from build123d import *

# Parameters (mm, degrees)
SKETCH_1_W      = 83.5
SKETCH_1_H      = 83.5
SKETCH_1_W_2    = 77.5
SKETCH_1_H_2    = 77.5
EXTRUDE_1_DEPTH = 20
CHAMFER_1_SIZE  = 1.5
SKETCH_2_W      = 83.5
SKETCH_2_H      = 83.5
EXTRUDE_2_DEPTH = 3


with BuildPart() as part:
    # Эскиз1 → Бобышка-Вытянуть1 (new body)
    with BuildSketch(Plane.XY):
        with Locations((38.75, 38.75)):
            Rectangle(SKETCH_1_W, SKETCH_1_H)
        with Locations((38.75, 38.75)):
            Rectangle(SKETCH_1_W_2, SKETCH_1_H_2, mode=Mode.SUBTRACT)
    extrude(amount=EXTRUDE_1_DEPTH)

    # Фаска1
    chamfer_1_edges = [part.edges().sort_by_distance(p)[0] for p in [
        (0, 38.75, 0),
        (38.75, 0, 0),
        (77.5, 38.75, 0),
        (38.75, 77.5, 0),
    ]]
    chamfer(chamfer_1_edges, length=CHAMFER_1_SIZE)

    # Эскиз2 → Бобышка-Вытянуть2 (add)
    with BuildSketch(Plane.XY.offset(20)):
        with Locations((38.75, 38.75)):
            Rectangle(SKETCH_2_W, SKETCH_2_H)
    extrude(amount=EXTRUDE_2_DEPTH)


solid = part.part
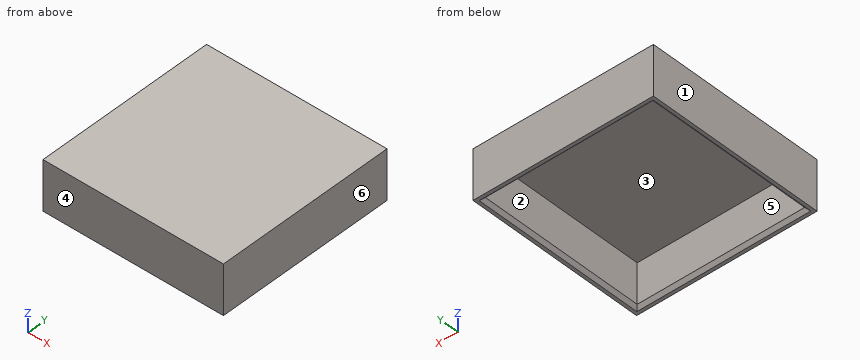
Input: part model. Units: mm. Frame: model coordinates. Face numbers are marked on the shaded views. A direction names the side the tool comes from. Coordinates: 2 decimals unless noted, no trailing zeros. Order: outer loops, then holes, each group sorted by start corner. A loop starts at its lowest first (then second) coordinate and runs counter-clockwise, first axis right, second up. Notation, with made-up numbers: M 29.5,56.25 L 50.5,56.25 A19 ccw 50.5,66.25 Z; hole C -37.75,30.5 d1. An arc over 180 degrees is marked long. Answer in a Markdown table with one row per item.
(1) Section query B-B, the plane z = 15.25. Output: boundary loops of the cut face in (x, y), plus the area to 3 significant figures.
Numbers:
| item | result |
|---|---|
| outline | M -3,-3 L 80.5,-3 L 80.5,80.5 L -3,80.5 Z; hole M 0,0 L 77.5,0 L 77.5,77.5 L 0,77.5 Z |
| area | 966 mm^2 |
(2) Contact query for a flat-ended pin moving along its axis: pin 1 Ø23 at (x, y) = (36, 52.5) entering from -Z. Output: stop coordinate, or through.
Numbers:
| item | result |
|---|---|
| pin 1 | stops at z = 20 |
(3) Draft query along Y for the marked faces 1, 2, 3 and 4. Return one class per face: pulls with the +Y half, pulls with the -Y half, needs draft (parallel to the pull), parting line crosses it, or undercut.
Numbers:
| item | result |
|---|---|
| face 1 | needs draft |
| face 2 | undercut |
| face 3 | undercut |
| face 4 | pulls with the -Y half |
(4) Section query A-A, the plane y = 5.5. Output: boundary loops of the cut face in (x, z).
Numbers:
| item | result |
|---|---|
| outline | M -3,0 L -1.5,0 L 0,1.5 L 0,20 L 77.5,20 L 77.5,1.5 L 79,0 L 80.5,0 L 80.5,23 L -3,23 Z |
(5) Access query for the marked faces 5 and 6. Directions: +Z, -Z, +X, -X, +Y, -Y. A direction counts if a zero-diameter tool reaches every point of the face in a straight line with its end or side. Return the directions, or none.
Numbers:
| item | result |
|---|---|
| face 5 | -Z |
| face 6 | +Z, -Z, +X, +Y, -Y |
(6) Material intervals for line 1 (Y direction, x = 45.5, z = 2.5); line 2 (Z direction, x = 45, y = 38), sorted ascending. Write a range as [from, to].
Numbers:
| item | result |
|---|---|
| line 1 | y = [-3, 0], [77.5, 80.5] |
| line 2 | z = [20, 23] |
